```python
from build123d import *

# Parameters (mm, degrees)
ESBO_O1_W                  = 32
ESBO_O1_H                  = 25
RESSALTO_EXTRUS_O1_DEPTH   = 3
PERFIL_CORTE_W             = 23
PERFIL_CORTE_H             = 12.4
CORTE_PRINCIPAL_DEPTH      = 81.646945091
FURO_DE_DI_METRO_3_0_3_1_D = 3
ESBO_O6_W                  = 3
ESBO_O6_H                  = 5
CORTE_EXTRUS_O2_DEPTH      = 81.150651679
FILETE1_R                  = 4


with BuildPart() as part:
    # Esboço1 → Ressalto-extrusão1 (new body)
    with BuildSketch(Plane(origin=(0, 0, 0), x_dir=(1, 0, 0), z_dir=(0, 1, 0))):
        Rectangle(ESBO_O1_W, ESBO_O1_H)
    extrude(amount=RESSALTO_EXTRUS_O1_DEPTH)

    # Perfil Corte → Corte Principal (cut, through all)
    with BuildSketch(Plane(origin=(-56.229726339, 3, 23.246277925), x_dir=(1, 0, 0), z_dir=(0, 1, 0))):
        with Locations((57.229726339, 23.246277925)):
            Rectangle(PERFIL_CORTE_W, PERFIL_CORTE_H)
    extrude(amount=-CORTE_PRINCIPAL_DEPTH, mode=Mode.SUBTRACT)

    # Furo de diâmetro Ø3.0 (3)1 (through all)
    with Locations(Plane(origin=(-54.773419901, 3, 25), x_dir=(1, 0, 0), z_dir=(0, 1, 0))):
        with Locations((55.773419901, 35), (55.773419901, 15)):
            Hole(FURO_DE_DI_METRO_3_0_3_1_D / 2)

    # Esboço6 → Corte-extrusão2 (cut, through all)
    with BuildSketch(Plane(origin=(-54.773419901, 3, 25), x_dir=(1, 0, 0), z_dir=(0, 1, 0))):
        with Locations((42.773419901, 25)):
            Rectangle(ESBO_O6_W, ESBO_O6_H)
    extrude(amount=-CORTE_EXTRUS_O2_DEPTH, mode=Mode.SUBTRACT)

    # Filete1
    filete1_edges = [part.edges().sort_by_distance(p)[0] for p in [
        (16, 1.5, 12.5),
        (-16, 1.5, 12.5),
        (-16, 1.5, -12.5),
        (16, 1.5, -12.5),
    ]]
    fillet(filete1_edges, radius=FILETE1_R)


solid = part.part
```
Input: part model. Units: mm. Frame: model coordinates. A direction names the side the tool comes from. Give positions to 0.01 mm unless a question says otherwise; leave off trailing zeros. Order: outer loops, then holes, each group sorted by start corner. A loop starts at its lowest first (then second) coordinate and runs counter-clockwise, first axis right, second up. Notation, with made-up numbers: M 23.5,21.25 L 36.5,21.25 A24 ccw 36.5,48.25 Z; hole C 30.25,73 d11. An arc over 180 degrees is marked long. Return JSON: item names as keys, results as strings.
Item 1: Ray query, probe 1 along Z at (x, y) = (1, 1.75); probe 2 along Z at (x, y) = (-11.5, 2.05); probe 3 along Z at (x, y) = (-6, 1.05). Return the intervals inside material, ascending.
Solutions:
{"probe 1": "-12.5 to -11.5, -8.5 to -6.2, 6.2 to 8.5, 11.5 to 12.5", "probe 2": "-12.5 to -2.5, 2.5 to 12.5", "probe 3": "-12.5 to -6.2, 6.2 to 12.5"}
Item 2: Pull-direction query (Z, two-part tool) for faces 1 (the flat face through (12.5, 2, 0)), 2 (the flat face through (-0.2, 0, -8.5)), 3 (the cylindrical face through (-14.859, 1.521, 11.297)); classes: +Z half, -Z half, draft (parallel to the pull), parting line (faces both ways), or undercut.
Solutions:
{"face 1": "undercut", "face 2": "draft", "face 3": "+Z half"}
Item 3: Cut plane C-C (y = 1.95). Return loops of the section in (x, z), then the cut area to 3 significant figures.
Solutions:
{"outline": "M -16,-8.5 A4 ccw -12,-12.5 L 12,-12.5 A4 ccw 16,-8.5 L 16,8.5 A4 ccw 12,12.5 L -12,12.5 A4 ccw -16,8.5 Z; hole M -13.5,-2.5 L -10.5,-2.5 L -10.5,-6.2 L 12.5,-6.2 L 12.5,6.2 L -10.5,6.2 L -10.5,2.5 L -13.5,2.5 Z; hole C 1,-10 d3; hole C 1,10 d3", "area": "472 mm^2"}
Item 4: Access query for faces 4 (the flat face through (16, 1, 0)), 5 (the flat face through (-12, 2, 2.5)). Directions: +Z, -Z, +X, -X, +Y, -Y. A direction counts if a zero-diameter tool reaches every point of the face in a straight line with its end or side. Return the directions, or none.
Solutions:
{"face 4": "+Z, -Z, +X, +Y, -Y", "face 5": "+Y, -Y"}
Item 5: Cut plane A-A (z = 5.75). Return loops of the section in (x, y).
Solutions:
{"outline": "M -16,0 L -10.5,0 L -10.5,3 L -16,3 Z; M 12.5,0 L 16,0 L 16,3 L 12.5,3 Z"}
Item 6: Cut plane B-B (x = -1.5). Return loops of the section in (y, z), then the cut area to 3 significant figures.
Solutions:
{"outline": "M 0,-12.5 L 3,-12.5 L 3,-6.2 L 0,-6.2 Z; M 0,6.2 L 3,6.2 L 3,12.5 L 0,12.5 Z", "area": "37.8 mm^2"}
